from build123d import *

# Parameters (mm, degrees)
SKETCH1_R           = 4.7625
SKETCH1_R_2         = 3.175
SKETCH1_R_3         = 4
BOSS_EXTRUDE1_DEPTH = 12.7
BOSS_EXTRUDE2_DEPTH = 0.889
SKETCH1_6_R         = 3.175
CUT_EXTRUDE1_DEPTH  = 6.477
SKETCH1_7_R         = 4
CUT_EXTRUDE2_DEPTH  = 8.89
CUT_EXTRUDE3_DEPTH  = 8.89
FILLET1_R           = 3.81
FILLET2_R           = 3.175
FILLET3_R           = 12.7


with BuildPart() as part:
    # Sketch1 → Boss-Extrude1 (new, symmetric)
    with BuildSketch(Plane(origin=(0, 0, 0), x_dir=(0, 1, 0), z_dir=(0, 0, 1))):
        with BuildLine():
            Line((21.356021011, 21.792976878), (37.358021011, 102.945465221))
            ThreePointArc((37.358021011, 102.945465221), (37.070944625, 107.078516049), (34.740471159, 110.503923386))
            Line((34.740471159, 110.503923386), (5.831671261, 135.319049463))
            ThreePointArc((5.831671261, 135.319049463), (-1.978401206, 136.605306542), (-6.716685754, 130.264932046))
            Line((-6.716685754, 130.264932046), (-14.212594445, 52.146935376))
            Line((-14.212594445, 52.146935376), (-7.560895503, -0.947237667))
            ThreePointArc((-7.560895503, -0.947237667), (-1.565846257, -7.457380606), (6.54135972, -3.908326114))
            Line((6.54135972, -3.908326114), (20.382390084, 19.257386231))
            ThreePointArc((20.382390084, 19.257386231), (20.978466311, 20.483226967), (21.356021011, 21.792976878))
        make_face()
        with Locations(Location((0, 0, 0), (0, 0, 90))):
            Circle(SKETCH1_R, mode=Mode.SUBTRACT)
        with Locations(Location((29.570473709, 104.48104761, 0), (0, 0, 90))):
            Circle(SKETCH1_R_2, mode=Mode.SUBTRACT)
        with Locations(Location((0.868473709, 129.537088718, 0), (0, 0, 90))):
            Circle(SKETCH1_R_3, mode=Mode.SUBTRACT)
        with Locations(Location((13.568473709, 23.328559267, 0), (0, 0, 90))):
            Circle(SKETCH1_R_2, mode=Mode.SUBTRACT)
        with BuildLine():
            Line((-2.479054789, 111.757088718), (11.028473709, 111.757088718))
            ThreePointArc((11.028473709, 111.757088718), (13.722550546, 110.641165554), (14.838473709, 107.947088718))
            Line((14.838473709, 107.947088718), (14.838473709, 89.9005863))
            ThreePointArc((14.838473709, 89.9005863), (14.417020328, 87.40152116), (13.199280383, 85.178896821))
            Line((13.199280383, 85.178896821), (-3.47332856, 64.060258828))
            ThreePointArc((-3.47332856, 64.060258828), (-7.883928971, 62.885691248), (-10.256311628, 66.785025232))
            Line((-10.256311628, 66.785025232), (-6.271634521, 108.311010382))
            ThreePointArc((-6.271634521, 108.311010382), (-5.041237302, 110.766897358), (-2.479054789, 111.757088718))
        make_face(mode=Mode.SUBTRACT)
        with BuildLine():
            Line((15.923267524, 85.759892349), (-9.835366262, 53.132289554))
            ThreePointArc((-9.835366262, 53.132289554), (-10.649296851, 50.563734965), (-9.560561043, 48.099062569))
            Line((-9.560561043, 48.099062569), (6.65017035, 31.626182714))
            ThreePointArc((6.65017035, 31.626182714), (8.557460112, 30.575295213), (10.728808005, 30.740725275))
            ThreePointArc((10.728808005, 30.740725275), (13.427097985, 31.264800137), (16.14234173, 30.837161644))
            ThreePointArc((16.14234173, 30.837161644), (19.280612759, 31.140473092), (21.115821085, 33.704211238))
            Line((21.115821085, 33.704211238), (30.769524141, 82.661968063))
            ThreePointArc((30.769524141, 82.661968063), (29.974660714, 85.818533808), (27.031501436, 87.20904761))
            Line((27.031501436, 87.20904761), (18.91367086, 87.20904761))
            ThreePointArc((18.91367086, 87.20904761), (17.252153249, 86.827671128), (15.923267524, 85.759892349))
        make_face(mode=Mode.SUBTRACT)
        with BuildLine():
            Line((-10.493663341, 36.765273562), (-7.837469994, 15.563413639))
            ThreePointArc((-7.837469994, 15.563413639), (-4.796024243, 12.29938936), (-0.741270636, 14.160362208))
            Line((-0.741270636, 14.160362208), (5.907210919, 25.907078618))
            ThreePointArc((5.907210919, 25.907078618), (6.36872877, 28.282081545), (5.30705743, 30.456131128))
            Line((5.30705743, 30.456131128), (-3.997617473, 39.911274641))
            ThreePointArc((-3.997617473, 39.911274641), (-8.373880181, 40.667929158), (-10.493663341, 36.765273562))
        make_face(mode=Mode.SUBTRACT)
    extrude(amount=BOSS_EXTRUDE1_DEPTH, both=True)

    # Sketch1_5 → Boss-Extrude2 (add, symmetric)
    with BuildSketch(Plane(origin=(0, 0, 0), x_dir=(0, 1, 0), z_dir=(0, 0, 1))):
        with BuildLine():
            Line((11.028473709, 111.757088718), (-2.479054789, 111.757088718))
            ThreePointArc((-2.479054789, 111.757088718), (-5.041237302, 110.766897358), (-6.271634521, 108.311010382))
            Line((-6.271634521, 108.311010382), (-10.256311628, 66.785025232))
            ThreePointArc((-10.256311628, 66.785025232), (-7.883928971, 62.885691248), (-3.47332856, 64.060258828))
            Line((-3.47332856, 64.060258828), (13.199280383, 85.178896821))
            ThreePointArc((13.199280383, 85.178896821), (14.417020328, 87.40152116), (14.838473709, 89.9005863))
            Line((14.838473709, 89.9005863), (14.838473709, 107.947088718))
            ThreePointArc((14.838473709, 107.947088718), (13.722550546, 110.641165554), (11.028473709, 111.757088718))
        make_face()
        with BuildLine():
            ThreePointArc((18.91367086, 87.20904761), (17.252153249, 86.827671128), (15.923267524, 85.759892349))
            Line((15.923267524, 85.759892349), (-9.835366262, 53.132289554))
            ThreePointArc((-9.835366262, 53.132289554), (-10.649296851, 50.563734965), (-9.560561043, 48.099062569))
            Line((-9.560561043, 48.099062569), (6.65017035, 31.626182714))
            ThreePointArc((6.65017035, 31.626182714), (8.557460112, 30.575295213), (10.728808005, 30.740725275))
            ThreePointArc((10.728808005, 30.740725275), (13.427097985, 31.264800137), (16.14234173, 30.837161644))
            ThreePointArc((16.14234173, 30.837161644), (19.280612759, 31.140473092), (21.115821085, 33.704211238))
            Line((21.115821085, 33.704211238), (30.769524141, 82.661968063))
            ThreePointArc((30.769524141, 82.661968063), (29.974660714, 85.818533808), (27.031501436, 87.20904761))
            Line((27.031501436, 87.20904761), (18.91367086, 87.20904761))
        make_face()
        with BuildLine():
            ThreePointArc((-3.997617473, 39.911274641), (-8.373880181, 40.667929158), (-10.493663341, 36.765273562))
            Line((-10.493663341, 36.765273562), (-7.837469994, 15.563413639))
            ThreePointArc((-7.837469994, 15.563413639), (-4.796024243, 12.29938936), (-0.741270636, 14.160362208))
            Line((-0.741270636, 14.160362208), (5.907210919, 25.907078618))
            ThreePointArc((5.907210919, 25.907078618), (6.36872877, 28.282081545), (5.30705743, 30.456131128))
            Line((5.30705743, 30.456131128), (-3.997617473, 39.911274641))
        make_face()
    extrude(amount=BOSS_EXTRUDE2_DEPTH, both=True)

    # Sketch1_6 → Cut-Extrude1 (cut, symmetric)
    with BuildSketch(Plane(origin=(0, 0, 0), x_dir=(0, 1, 0), z_dir=(0, 0, 1))):
        with BuildLine():
            Line((16.870473709, 89.24104761), (34.655724444, 89.24104761))
            Line((34.655724444, 89.24104761), (37.358021011, 102.945465221))
            ThreePointArc((37.358021011, 102.945465221), (37.070944625, 107.078516049), (34.740471159, 110.503923386))
            Line((34.740471159, 110.503923386), (16.870473709, 125.843413136))
            Line((16.870473709, 125.843413136), (16.870473709, 89.24104761))
        make_face()
        with Locations(Location((29.570473709, 104.48104761, 0), (0, 0, 90))):
            Circle(SKETCH1_6_R, mode=Mode.SUBTRACT)
    extrude(amount=CUT_EXTRUDE1_DEPTH, both=True, mode=Mode.SUBTRACT)

    # Sketch1_7 → Cut-Extrude2 (cut, symmetric)
    with BuildSketch(Plane(origin=(0, 0, 0), x_dir=(0, 1, 0), z_dir=(0, 0, 1))):
        with BuildLine():
            Line((14.838473709, 114.297088718), (14.838473709, 127.587668738))
            Line((14.838473709, 127.587668738), (5.831671261, 135.319049463))
            ThreePointArc((5.831671261, 135.319049463), (-1.978401206, 136.605306542), (-6.716685754, 130.264932046))
            Line((-6.716685754, 130.264932046), (-8.248899849, 114.297088718))
            Line((-8.248899849, 114.297088718), (14.838473709, 114.297088718))
        make_face()
        with Locations(Location((0.868473709, 129.537088718, 0), (0, 0, 90))):
            Circle(SKETCH1_7_R, mode=Mode.SUBTRACT)
    extrude(amount=CUT_EXTRUDE2_DEPTH, both=True, mode=Mode.SUBTRACT)

    # Sketch1_9 → Cut-Extrude3 (cut, symmetric)
    with BuildSketch(Plane(origin=(0, 0, 0), x_dir=(0, 1, 0), z_dir=(0, 0, 1))):
        Polygon((10.542747735, 2.788791174), (16.405901968, 12.601943868), (4.298278893, 19.454693681), (-1.330811933, 9.509064286), align=None)
    extrude(amount=CUT_EXTRUDE3_DEPTH, both=True, mode=Mode.SUBTRACT)

    # Fillet1
    fillet1_edges = [part.edges().sort_by_distance(p)[0] for p in [
        (-107.542230373, 16.870473709, 6.477),
        (-107.542230373, 16.870473709, -6.477),
        (-120.942378728, 14.838473709, -8.89),
        (-120.942378728, 14.838473709, 8.89),
        (-16.028318774, 10.352090431, 8.89),
        (-6.14892773, 4.605967901, -8.89),
        (-16.028318774, 10.352090431, -8.89),
        (-6.14892773, 4.605967901, 8.89),
    ]]
    fillet(fillet1_edges, radius=FILLET1_R)

    # Fillet2
    fillet2_edges = [part.edges().sort_by_distance(p)[0] for p in [
        (-89.24104761, 27.668099077, 6.477),
        (-89.24104761, 16.870473709, 0),
        (-89.24104761, 27.668099077, -6.477),
        (-89.24104761, 17.986396873, -5.361076836),
        (-89.24104761, 17.986396873, 5.361076836),
        (-114.297088718, 14.838473709, 0),
        (-114.297088718, 1.38978693, 8.89),
        (-114.297088718, 1.38978693, -8.89),
        (-114.297088718, 13.722550546, -7.774076836),
        (-114.297088718, 13.722550546, 7.774076836),
    ]]
    fillet(fillet2_edges, radius=FILLET2_R)

    # Fillet3
    fillet3_edges = [part.edges().sort_by_distance(p)[0] for p in [
        (-52.146935376, -14.212594445, 0),
    ]]
    fillet(fillet3_edges, radius=FILLET3_R)


solid = part.part
Input: part model. Units: mm. Frame: model coordinates. A direction names the side the tool comes from. Give positions to 0.01 mm unless a question says otherwise; leave off trailing zeros. Write each loop counter-clockwise with the first axis right and the second up, starting at its lowest first coordinate (ties: lowest second). Pieces come first, ordered by that corner, then holes. Notation, with made-up numbers: M 24.25,32.25 L 34.25,32.25 A7 cw 34.25,44.25 Z; hole C 70,-7.5 d6. An arc over 180 degrees is marked long. Use one line per item in the form item = value.
1. Cut plane A-A on x = -95. Return loops of the section in (y, z).
Outcome:
outline = M -10.1,-12.7 L -7.55,-12.7 L -7.55,-0.89 L 14.84,-0.89 L 14.84,-12.7 L 35.79,-12.7 L 35.79,-6.48 L 20.68,-6.48 A3.81 cw 16.87,-2.67 L 16.87,2.67 A3.81 cw 20.68,6.48 L 35.79,6.48 L 35.79,12.7 L 14.84,12.7 L 14.84,0.89 L -7.55,0.89 L -7.55,12.7 L -10.1,12.7 Z
2. Cut plane B-B on x = -80.5. Return loops of the section in (y, z), and give its area (3 significant figures).
Outcome:
outline = M -11.49,-12.7 L -8.94,-12.7 L -8.94,-0.89 L 9.51,-0.89 L 9.51,-12.7 L 11.77,-12.7 L 11.77,-0.89 L 30.34,-0.89 L 30.34,-12.7 L 32.93,-12.7 L 32.93,12.7 L 30.34,12.7 L 30.34,0.89 L 11.77,0.89 L 11.77,12.7 L 9.51,12.7 L 9.51,0.89 L -8.94,0.89 L -8.94,12.7 L -11.49,12.7 Z
area = 254 mm²
3. Mould query, pull axis Y, two halves, no side actions, for faces 4 (the face through (-70, 2, -12.7)), 5 (the face through (-107.02, 37.09, -9.54)), 6 (the face through (-110.671, 13.693, -6.712)). Classes: released by +Y, released by -Y, zero draft, split by the parting line, or undercut.
Outcome:
face_4 = zero draft
face_5 = released by +Y
face_6 = undercut
4. First-contact query: P1, Ø1.5, axis at x = -40, z = 0.5, coming from the -Y side; P2, Ø11, axis at x = 0, y = 0, coming from the -Z side; P3, Ø13, axis at x = -101, z = -4.5, coming from the -Y side; P4, Ø11, axis at x = -120.5, z = -2.5, coming from the -Y side. Flat tips, straight axial feed; report the tip coordinate or a pass-through.
Outcome:
P1 = -12.78
P2 = -12.7
P3 = -10.15
P4 = 13.48
5. Reachability of faces 1 (the face through (-87.44, 14.43, -6.88)), 2 (the face through (-108.896, 18.016, -5.391)), 3 (the face through (-62.86, -7.82, 6.88)) from +Z, -Z, +X, -X, +Y, -Y: full face, straight path, thin tool, end or side. Return the list, or none.
Outcome:
face_1 = -Z
face_2 = -X, +Y
face_3 = +Z
6. Ray query, L1, parallel to Z at x = -112, y = 29; L2, parallel to X at y = -3, z = -3.5; L3, parallel to X at y = 15, z = -2.5. Return the intervals inside material, ascending.
Outcome:
L1 = -12.7 to -6.48, 6.48 to 12.7
L2 = -114.3 to -111.72, -64.66 to -61.79, -41.43 to -38.9, -12.38 to -3.7, 3.7 to 7
L3 = -127.45 to -84.59, -31.14 to -26.16, -20.49 to -13.4
